Input: part model. Units: mm. Frame: model coordinates. A direction names the side the tool comes from. Coordinates: 2 decimals unless noted, no trailing zeros. Write each loop counter-clockwise with the first axis right and the second up, starting at its lowest first coordinate (ties: lowest second). Pieces come first, ordered by that corner, then holes. Notation, with made-up numbers: (66, 67.25) - (78, 67.25) arc R22 cw to (78, 81.25) - close; hole circle Ø6 at (68, 49.25). An arc over 180 degrees is marked (long way). Use a Markdown table: item, result. Add a question column.
Q1. Section query A-A (x = 42). Return the cut outline in (y, z), then the cut area to 3 significant figures.
Q2. Section query C-C (x = -45). Return the cut outline in (y, z), then the cut area to 3 significant figures.
Q3. Mould query, pull axis X, two halves, no side actions, for faces 4 (the face through (51.6, -11.14, 2.54)), 5 (the face through (0.01, 22.59, 2.46)), 6 (the face through (0, 2, 2)). Classes: released by +X, released by -X, zero draft, split by the parting line, or undercut.
Q4. Material intervals for probe 1 along Y at (x, z) = (-11, 2.15); probe 2 along Y at (x, z) = (15.5, 2.8), sorted ascending. Write a range as from..to.
Q5. Set-up query: faces 1 (the face through (-51.64, -11.1, 2.54)), 2 (the face through (-37.5, -8, 2)), 3 (the face through (-4.375, 11, 2)). Return all of +Z, -Z, +X, -X, +Y, -Y with unobstructed straight access to the full face (end or side cutting, diameter ignored); none if empty.
Q6. Section query B-B (z = 1.55). Give the number of separate pieces and of enclosed holes in the cut face, then the cut area to 3 significant figures.
from build123d import *

# Parameters (mm, degrees)
F0_R     = 3.9
F1_DEPTH = 5
F2_DEPTH = 25
F3_R     = 1
F4_R     = 3


with BuildPart() as f1:
    # F0 (on Top) → F1 (new body)
    with BuildSketch(Plane.XY):
        with BuildLine():
            ThreePointArc((-46.9082644116, 7.2531735768), (-43.1416684259, 7.2661271501), (-39.8437820891, 5.4464132101))
            Line((-39.8437820891, 5.4464132101), (-10.8327285679, 15.0306360845))
            ThreePointArc((-10.8327285679, 15.0306360845), (-8.1342763091, 14.6134381435), (-6.8916598566, 12.1820593029))
            Line((-6.8916598566, 12.1820593029), (-6.8916598566, 4.4145286559))
            ThreePointArc((-6.8916598566, 4.4145286559), (-7.6005216796, 2.4778599043), (-9.3921170923, 1.4564115138))
            Line((-9.3921170923, 1.4564115138), (-37.5, -3.2902191476))
            Line((-37.5, -3.2902191476), (-37.5, -6.332695009))
            Line((-37.5, -6.332695009), (-0.4995427643, -0.0843587192))
            ThreePointArc((-0.4995427643, -0.0843587192), (0, -0.0424758613), (0.4995427643, -0.0843587192))
            Line((0.4995427643, -0.0843587192), (37.5, -6.332695009))
            Line((37.5, -6.332695009), (37.5, -3.2902191476))
            Line((37.5, -3.2902191476), (9.3921170923, 1.4564115138))
            ThreePointArc((9.3921170923, 1.4564115138), (7.6005216796, 2.4778599043), (6.8916598566, 4.4145286559))
            Line((6.8916598566, 4.4145286559), (6.8916598566, 12.1820593029))
            ThreePointArc((6.8916598566, 12.1820593029), (8.1342763091, 14.6134381435), (10.8327285679, 15.0306360845))
            Line((10.8327285679, 15.0306360845), (39.8437820891, 5.4464132101))
            ThreePointArc((39.8437820891, 5.4464132101), (43.1416684259, 7.2661271501), (46.9082644116, 7.2531735768))
            Line((46.9082644116, 7.2531735768), (0.9410687113, 22.4391042836))
            ThreePointArc((0.9410687113, 22.4391042836), (0, 22.590527502), (-0.9410687113, 22.4391042836))
            Line((-0.9410687113, 22.4391042836), (-46.9082644116, 7.2531735768))
        make_face()
        with BuildLine():
            ThreePointArc((-4.375, 16.375), (0, 20.75), (4.375, 16.375))
            Line((4.375, 16.375), (4.375, 6.375))
            ThreePointArc((4.375, 6.375), (0, 2), (-4.375, 6.375))
            Line((-4.375, 6.375), (-4.375, 16.375))
        make_face(mode=Mode.SUBTRACT)
        with BuildLine():
            Line((-37.5, -3.2902191476), (-38.3305275597, -3.4304718872))
            ThreePointArc((-38.3305275597, -3.4304718872), (-40.4438234256, -5.9574537365), (-43.4360893176, -7.3351334942))
            Line((-43.4360893176, -7.3351334942), (-37.5, -6.332695009))
            Line((-37.5, -6.332695009), (-37.5, -3.2902191476))
        make_face()
        with BuildLine():
            ThreePointArc((-38.3305275597, -3.4304718872), (-37.7105883879, -1.7647884715), (-37.5, 0))
            ThreePointArc((-37.5, 0), (-38.110818832, 2.9646556012), (-39.8437820891, 5.4464132101))
            ThreePointArc((-39.8437820891, 5.4464132101), (-43.1416684259, 7.2661271501), (-46.9082644116, 7.2531735768))
            ThreePointArc((-46.9082644116, 7.2531735768), (-50.9397804289, 4.5791929919), (-52.5, 0))
            ThreePointArc((-52.5, 0), (-49.7180859404, -5.8300656136), (-43.4360893176, -7.3351334942))
            ThreePointArc((-43.4360893176, -7.3351334942), (-40.4438234256, -5.9574537365), (-38.3305275597, -3.4304718872))
        make_face()
        with Locations((-45, 0)):
            Circle(F0_R, mode=Mode.SUBTRACT)
        with BuildLine():
            ThreePointArc((52.5, 0), (50.9397804289, 4.5791929919), (46.9082644116, 7.2531735768))
            ThreePointArc((46.9082644116, 7.2531735768), (43.1416684259, 7.2661271501), (39.8437820891, 5.4464132101))
            ThreePointArc((39.8437820891, 5.4464132101), (38.110818832, 2.9646556012), (37.5, 0))
            Line((37.5, 0), (41.1, 0))
            ThreePointArc((41.1, 0), (45, 3.9), (48.9, 0))
            Line((48.9, 0), (52.5, 0))
        make_face()
        with BuildLine():
            ThreePointArc((43.4360893176, -7.3351334942), (49.7180859404, -5.8300656136), (52.5, 0))
            Line((52.5, 0), (48.9, 0))
            ThreePointArc((48.9, 0), (45, -3.9), (41.1, 0))
            Line((41.1, 0), (37.5, 0))
            ThreePointArc((37.5, 0), (37.7105883879, -1.7647884715), (38.3305275597, -3.4304718872))
            ThreePointArc((38.3305275597, -3.4304718872), (40.4438234256, -5.9574537365), (43.4360893176, -7.3351334942))
        make_face()
        with BuildLine():
            Line((37.5, -3.2902191476), (37.5, -6.332695009))
            Line((37.5, -6.332695009), (43.4360893176, -7.3351334942))
            ThreePointArc((43.4360893176, -7.3351334942), (40.4438234256, -5.9574537365), (38.3305275597, -3.4304718872))
            Line((38.3305275597, -3.4304718872), (37.5, -3.2902191476))
        make_face()
        with BuildLine():
            Line((43.4360893176, -7.3351334942), (37.5, -6.332695009))
            Line((37.5, -6.332695009), (37.5, -12))
            Line((37.5, -12), (52.5, -12))
            Line((52.5, -12), (52.5, 0))
            ThreePointArc((52.5, 0), (49.7180859404, -5.8300656136), (43.4360893176, -7.3351334942))
        make_face()
        with BuildLine():
            Line((-37.5, -6.332695009), (-43.4360893176, -7.3351334942))
            ThreePointArc((-43.4360893176, -7.3351334942), (-49.7180859404, -5.8300656136), (-52.5, 0))
            Line((-52.5, 0), (-52.5, -12))
            Line((-52.5, -12), (-37.5, -12))
            Line((-37.5, -12), (-37.5, -6.332695009))
        make_face()
    extrude(amount=F1_DEPTH)

    # F0 (on Top) → F2 (cut)
    with BuildSketch(Plane.XY):
        with Locations((-45, 0)):
            Circle(F0_R)
        with BuildLine():
            Line((41.1, 0), (48.9, 0))
            ThreePointArc((48.9, 0), (45, 3.9), (41.1, 0))
        make_face()
        with BuildLine():
            ThreePointArc((41.1, 0), (45, -3.9), (48.9, 0))
            Line((48.9, 0), (41.1, 0))
        make_face()
    extrude(amount=F2_DEPTH, mode=Mode.SUBTRACT)

    # F3
    f3_edges = [f1.edges().sort_by_distance(p)[0] for p in [
        (-39.843782, 5.446413, 2.5),
        (-38.330528, -3.430472, 2.5),
        (39.843782, 5.446413, 2.5),
        (38.330528, -3.430472, 2.5),
    ]]
    fillet(f3_edges, radius=F3_R)

    # F4
    f4_edges = [f1.edges().sort_by_distance(p)[0] for p in [
        (-52.5, -12, 2.5),
        (-37.5, -12, 2.5),
        (37.5, -12, 2.5),
        (52.5, -12, 2.5),
    ]]
    fillet(f4_edges, radius=F4_R)


solid = f1.part
Values follow:
| question | item | result |
|---|---|---|
| 1 | outline | (-12, 0) - (-2.49, 0) - (-2.49, 5) - (-12, 5) - close; (2.49, 0) - (8.87, 0) - (8.87, 5) - (2.49, 5) - close |
| 1 | area | 79.5 mm2 |
| 2 | outline | (-12, 0) - (-3.9, 0) - (-3.9, 5) - (-12, 5) - close; (3.9, 0) - (7.88, 0) - (7.88, 5) - (3.9, 5) - close |
| 2 | area | 60.4 mm2 |
| 3 | face 4 | released by +X |
| 3 | face 5 | split by the parting line |
| 3 | face 6 | undercut |
| 4 | probe 1 | -1.86..1.18, 14.98..19.12 |
| 4 | probe 2 | -2.62..0.42, 13.49..17.63 |
| 5 | face 1 | +Z, -Z, -X, -Y |
| 5 | face 2 | +Z, -Z, -Y |
| 5 | face 3 | +Z, -Z |
| 6 | separate pieces | 1 |
| 6 | enclosed holes | 5 |
| 6 | area | 1,080 mm2 |
